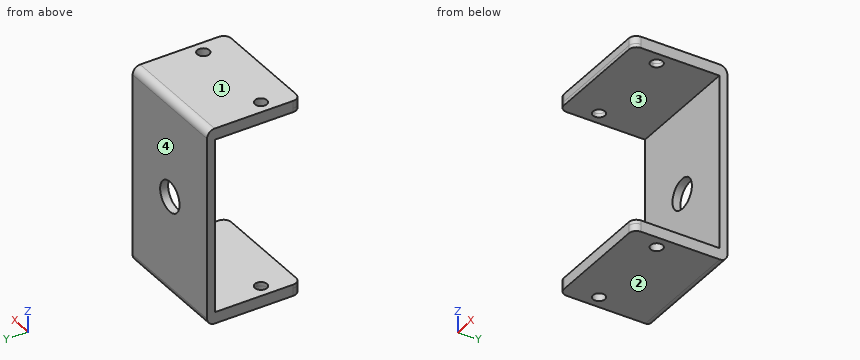
from build123d import *
from build123d.topology import SkipClean

# Parameters (mm, degrees)
SKETCH_1_W               = 30
SKETCH_1_H               = 65
EXTRUDE_1_DEPTH          = 48
SKETCH_2_R               = 1
CUT_EXTRUDE_1_DEPTH      = 48
EXTRUDE_2_DEPTH          = 5
EXTRUDE_2_DEPTH_BACK     = 53
SKETCH_3_R               = 3
CHAMFER_1_SIZE           = 2
FILLET_1_R               = 1
FILLET_2_R               = 1
SKETCH_6_R               = 1.6
CUT_EXTRUDE_3_DEPTH      = 76
EXTRUDE_3_DEPTH          = 50
EXTRUDE_3_DEPTH_BACK     = 2
SKETCH_7_W               = 30.741029275
SKETCH_7_H               = 24.773895079
SKETCH_7_R               = 1.6
CUT_EXTRUDE_START        = -30.741029275
CUT_EXTRUDE_4_DEPTH      = 30.741029275
CUT_EXTRUDE_5_DEPTH      = 50
CUT_EXTRUDE_5_DEPTH_BACK = 50
SKETCH_9_R               = 4
FILLET_3_R               = 2


# Read off the part's stored shape, not the designer's step: ｶｯﾄ - 押し出し4
with BuildPart() as part:
    # ｽｹｯﾁ1 → ﾎﾞｽ - 押し出し1 (new body)
    with BuildSketch(Plane.XY):
        with Locations((44.026916893, 39.150883092)):
            Rectangle(SKETCH_1_W, SKETCH_1_H)
    extrude(amount=EXTRUDE_1_DEPTH)

    # ｽｹｯﾁ2 → ｶｯﾄ - 押し出し1 (cut)
    with BuildSketch(Plane.XY):
        with Locations((56.026916893, 57.650883092)):
            Circle(SKETCH_2_R)
        with Locations((44.026916893, 57.650883092)):
            Circle(SKETCH_2_R)
        with Locations((56.023819064, 45.923533591)):
            Circle(SKETCH_2_R)
        with Locations((32.026916893, 57.650883092)):
            Circle(SKETCH_2_R)
        with Locations(Location((32.030014722, 45.923533591, 0), (0, 0, 180))):
            Circle(SKETCH_2_R)
    extrude(amount=CUT_EXTRUDE_1_DEPTH, mode=Mode.SUBTRACT)

    # ｽｹｯﾁ3 → ﾎﾞｽ - 押し出し2 (add, two sides: drawn at the far end of the back side and taken through both)
    with BuildSketch(Plane(origin=(0, 0, 0), x_dir=(-1, 0, 0), z_dir=(0, 0, -1)).offset(-EXTRUDE_2_DEPTH_BACK)):
        with Locations((-44.026916893, 18.650883092)):
            Circle(SKETCH_3_R)
    extrude(amount=EXTRUDE_2_DEPTH + EXTRUDE_2_DEPTH_BACK)

    # 面取り1
    chamfer_1_edges = [part.edges().sort_by_distance(p)[0] for p in [
        (29.026916893, 71.650883092, 24),
        (59.026916893, 71.650883092, 24),
        (59.026916893, 6.650883092, 24),
        (29.026916893, 6.650883092, 24),
    ]]
    chamfer(chamfer_1_edges, length=CHAMFER_1_SIZE)

    # ﾌｨﾚｯﾄ1
    fillet_1_edges = [part.edges().sort_by_distance(p)[0] for p in [
        (44.026916893, 6.650883092, 48),
        (29.026916893, 39.150883092, 48),
        (59.026916893, 39.150883092, 48),
        (44.026916893, 71.650883092, 48),
        (30.026916893, 70.650883092, 48),
        (58.026916893, 70.650883092, 48),
        (58.026916893, 7.650883092, 48),
        (30.026916893, 7.650883092, 48),
    ]]
    fillet(fillet_1_edges, radius=FILLET_1_R)

    # ﾌｨﾚｯﾄ2
    fillet_2_edges = [part.edges().sort_by_distance(p)[0] for p in [
        (44.026916893, 6.650883092, 0),
        (29.026916893, 39.150883092, 0),
        (44.026916893, 71.650883092, 0),
        (59.026916893, 39.150883092, 0),
        (30.026916893, 70.650883092, 0),
        (58.026916893, 70.650883092, 0),
        (58.026916893, 7.650883092, 0),
        (30.026916893, 7.650883092, 0),
    ]]
    fillet(fillet_2_edges, radius=FILLET_2_R)

    # ｽｹｯﾁ6 → ｶｯﾄ - 押し出し3 (cut)
    with BuildSketch(Plane(origin=(0, 0, 0), x_dir=(-1, 0, 0), z_dir=(0, 0, -1))):
        with Locations((-55.99912174, 57.606952707)):
            Circle(SKETCH_6_R)
        with Locations((-32.054712046, 57.694813478)):
            Circle(SKETCH_6_R)
        with Locations((-55.99912174, 45.879603206)):
            Circle(SKETCH_6_R)
        with Locations((-32.054712046, 45.967463976)):
            Circle(SKETCH_6_R)
    extrude(amount=-CUT_EXTRUDE_3_DEPTH, mode=Mode.SUBTRACT)

    # ｽｹｯﾁ7 → ﾎﾞｽ - 押し出し3 (add, two sides: drawn at the far end of the back side and taken through both)
    with SkipClean():  # the faces are left unmerged after this step: merging them gives an invalid solid
        with BuildSketch(Plane.XY.offset(-EXTRUDE_3_DEPTH_BACK)):
            with Locations((44.019576577, 61.733784516)):
                Rectangle(SKETCH_7_W, SKETCH_7_H)
            with Locations((32.054712046, 57.694813478)):
                Circle(SKETCH_7_R, mode=Mode.SUBTRACT)
            with Locations((55.99912174, 57.606952707)):
                Circle(SKETCH_7_R, mode=Mode.SUBTRACT)
        extrude(amount=EXTRUDE_3_DEPTH + EXTRUDE_3_DEPTH_BACK)

    # ｶｯﾄ - 押し出し4 outline → ｶｯﾄ - 押し出し4 (cut)
    with SkipClean():  # the faces are left unmerged after this step: merging them gives an invalid solid
        with BuildSketch(Plane(origin=(59.390091214, 0, 0), x_dir=(0, 0, -1), z_dir=(1, 0, 0)).offset(CUT_EXTRUDE_START)):
            Polygon((-1, 49.346836976), (-1, 72.013202711), (-47, 72.013202711), (-47, 49.346836976), (-48, 49.346836976), (-48, 45.206300999), (-57.188140565, 45.206300999), (-57.188140565, 1.456905632), (13.746291121, 1.456905632), (13.746291121, 49.346836976), align=None)
        extrude(amount=CUT_EXTRUDE_4_DEPTH, mode=Mode.SUBTRACT)

    # ｽｹｯﾁ9 → ｶｯﾄ - 押し出し5 (cut, two sides: drawn at the far end of the back side and taken through both)
    with SkipClean():  # the faces are left unmerged after this step: merging them gives an invalid solid
        with BuildSketch(Plane(origin=(0, 74.120732055, 0), x_dir=(1, 0, 0), z_dir=(0, 1, 0)).offset(-CUT_EXTRUDE_5_DEPTH_BACK)):
            with Locations(Location((44.019576577, -24, 0), (0, 0, 270))):
                Circle(SKETCH_9_R)
        extrude(amount=CUT_EXTRUDE_5_DEPTH + CUT_EXTRUDE_5_DEPTH_BACK, mode=Mode.SUBTRACT)

    # ﾌｨﾚｯﾄ3
    fillet_3_edges = [part.edges().sort_by_distance(p)[0] for p in [
        (28.649061939, 49.346836976, -0.5),
        (44.019576577, 74.120732055, -2),
        (59.390091214, 49.346836976, -0.5),
        (44.019576577, 74.120732055, 50),
        (59.390091214, 49.346836976, 49),
        (28.649061939, 49.346836976, 49),
    ]]
    fillet(fillet_3_edges, radius=FILLET_3_R)


solid = part.part
Input: part model. Units: mm. Frame: model coordinates. Face numbers are marked on the shaded views. Give positions to 0.01 mm unless a question says otherwise; leave off trailing zeros. Order: outer loops, then holes, each group sorted by start corner. A loop starts at its lowest first (then second) coordinate and runs counter-clockwise, first axis right, second up. Notation, with made-up numbers: (34, -36) -> (49, -36) arc R17 ccw to (49, -8) -> close; hole circle Ø3 at (15.25, 46.25). An arc over 180 degrees is marked (long way). Use one line per item in the form item = value.
1) Mould query, pull axis Z, two halves, no side actions, for the marked faces 1, 2, 3 and 4. Classes: pulls with the +Z half, pulls with the -Z half, needs draft (parallel to the pull), parting line crosses it, or undercut.
Response values:
face_1 = pulls with the +Z half
face_2 = pulls with the -Z half
face_3 = undercut
face_4 = needs draft
2) Section A-A, the plane x = 56. Return loops of the section in (y, z).
Response values:
outline = (49.35, -2) -> (56.01, -2) -> (56.01, 1) -> (49.35, 1) -> close; (49.35, 47) -> (56.01, 47) -> (56.01, 50) -> (49.35, 50) -> close; (59.21, -2) -> (72.12, -2) arc R2 ccw to (74.12, 0) -> (74.12, 48) arc R2 ccw to (72.12, 50) -> (59.21, 50) -> (59.21, 47) -> (72.01, 47) -> (72.01, 1) -> (59.21, 1) -> close
3) First-contact query: pin 1 Ø3 at (x, z) = (48.5, 9) entering from -Y; pin 2 Ø6.5 at (x, z) = (44.02, 24) entering from +Y. Flat tips, straight axial feed; report the tip coordinate or a pass-through.
Response values:
pin_1 = 72.01
pin_2 = through
4) Section D-D, the plane x = 36.5. Return loops of the section in (y, z), and give its area (3 significant figures).
Response values:
outline = (49.35, -2) -> (72.12, -2) arc R2 ccw to (74.12, 0) -> (74.12, 48) arc R2 ccw to (72.12, 50) -> (49.35, 50) -> (49.35, 47) -> (72.01, 47) -> (72.01, 1) -> (49.35, 1) -> close
area = 244 mm^2
5) Line query: probe 1 along Z at (x, y) = (37, 61.75); probe 2 along Y at (x, z) = (52, 22.5); probe 3 along Z at (x, y) = (57, 72.25). Output: solid intervals per line, ascending.
Response values:
probe_1 = -2 to 1, 47 to 50
probe_2 = 72.01 to 74.12
probe_3 = -2 to 50
6) Section B-B, the plane z = 24. Return loops of the section in (x, y), and give its area (3 significant figures).
Response values:
outline = (28.65, 72.01) -> (40.02, 72.01) -> (40.02, 74.12) -> (28.65, 74.12) -> close; (48.02, 72.01) -> (59.39, 72.01) -> (59.39, 74.12) -> (48.02, 74.12) -> close
area = 47.9 mm^2
7) Section C-C, the plane y = 65.5. Return loops of the section in (x, z), and give its area (3 significant figures).
Response values:
outline = (28.65, -2) -> (59.39, -2) -> (59.39, 1) -> (28.65, 1) -> close; (28.65, 47) -> (59.39, 47) -> (59.39, 50) -> (28.65, 50) -> close
area = 184 mm^2
